CAD build for the part. Positions are in the model's coordinates, mm. A direction names the side the tool comes from. Give positions to 0.01 mm unless a question says otherwise; leave off trailing zeros. Write each loop counter-clockwise with the first axis right and the second up, starting at its lowest first coordinate (ties: lowest second). Pieces come first, ordered by that corner, then holes. Notation, with made-up numbers: (46, 19.25) - (54, 19.25) arc R20 ccw to (54, 48.25) - close; hole circle Ø8 at (-4, -35). An arc over 180 degrees is marked (long way). Write item = value, one per line. Start each with the question number.
```python
from build123d import *

# Parameters (mm, degrees)
SKETCH_1_W             = 55.4
SKETCH_1_H             = 37.5
SKETCH_1_W_2           = 30
SKETCH_1_H_2           = 4
EXTRUDE_1_DEPTH        = 3
SKETCH_2_R             = 1.25
CUT_EXTRUDE_1_DEPTH    = 67.965737508
SKETCH_3_W             = 10
SKETCH_3_H             = 10.5
CUT_EXTRUDE_2_DEPTH    = 67.965737508
FILLET_2_R             = 1
FILLET_3_R             = 2
SKETCH_6_R             = 1.5
CUT_EXTRUDE_4_DEPTH    = 67.965737508
SKETCH_7_R             = 3
CUT_EXTRUDE_5_DEPTH    = 1.8
FILLET_4_R             = 8
SKETCH_10_W            = 31.4
SKETCH_10_H            = 23
CUT_EXTRUDE_6_DEPTH    = 10
FILLET_5_R             = 8
FILLET_6_R             = 2
HOLE_WIZARD_M3_1_D     = 2.5
HOLE_WIZARD_M3_1_DEPTH = 3
HOLE_WIZARD_M3_1_TIP   = 0.751075774


with BuildPart() as part:
    # 草图1 → 凸台-拉伸1 (new body)
    with BuildSketch(Plane(origin=(0, 0, 0), x_dir=(0, 0, -1), z_dir=(1, 0, 0))):
        with Locations((27.7, 18.75)):
            Rectangle(SKETCH_1_W, SKETCH_1_H)
        with Locations((27.7, 34)):
            Rectangle(SKETCH_1_W_2, SKETCH_1_H_2, mode=Mode.SUBTRACT)
    extrude(amount=EXTRUDE_1_DEPTH)

    # 草图2 → 切除-拉伸1 (cut, through all)
    with BuildSketch(Plane(origin=(3, 0, 0), x_dir=(0, 0, -1), z_dir=(1, 0, 0))):
        with Locations((5.2, 21)):
            Circle(SKETCH_2_R)
        with Locations((5.2, 2.5)):
            Circle(SKETCH_2_R)
        with Locations((50.2, 21)):
            Circle(SKETCH_2_R)
        with Locations((50.2, 2.5)):
            Circle(SKETCH_2_R)
    extrude(amount=-CUT_EXTRUDE_1_DEPTH, mode=Mode.SUBTRACT)

    # 草图3 → 切除-拉伸2 (cut, through all)
    with BuildSketch(Plane(origin=(3, 0, 0), x_dir=(0, 0, -1), z_dir=(1, 0, 0))):
        with Locations((5, 32.25)):
            Rectangle(SKETCH_3_W, SKETCH_3_H)
        with Locations((50.4, 32.25)):
            Rectangle(SKETCH_3_W, SKETCH_3_H)
    extrude(amount=-CUT_EXTRUDE_2_DEPTH, mode=Mode.SUBTRACT)

    # 圆角2
    fillet_2_edges = [part.edges().sort_by_distance(p)[0] for p in [
        (1.5, 36, -12.7),
        (1.5, 32, -12.7),
        (1.5, 32, -42.7),
        (1.5, 36, -42.7),
    ]]
    fillet(fillet_2_edges, radius=FILLET_2_R)

    # 圆角3
    fillet_3_edges = [part.edges().sort_by_distance(p)[0] for p in [
        (1.5, 37.5, -10),
        (1.5, 37.5, -45.4),
    ]]
    fillet(fillet_3_edges, radius=FILLET_3_R)

    # 草图6 → 切除-拉伸4 (cut, through all)
    with BuildSketch(Plane.ZY):
        with Locations((-47.4, 13.5)):
            Circle(SKETCH_6_R)
        with Locations((-8, 13.5)):
            Circle(SKETCH_6_R)
    extrude(amount=-CUT_EXTRUDE_4_DEPTH, mode=Mode.SUBTRACT)

    # 草图7 → 切除-拉伸5 (cut)
    with BuildSketch(Plane.ZY):
        with Locations((-47.4, 13.5)):
            Circle(SKETCH_7_R)
        with Locations((-8, 13.5)):
            Circle(SKETCH_7_R)
    extrude(amount=-CUT_EXTRUDE_5_DEPTH, mode=Mode.SUBTRACT)

    # 圆角4
    fillet_4_edges = [part.edges().sort_by_distance(p)[0] for p in [
        (1.5, 27, -10),
        (1.5, 27, -45.4),
    ]]
    fillet(fillet_4_edges, radius=FILLET_4_R)

    # 草图10 → 切除-拉伸6 (cut)
    with BuildSketch(Plane.ZY):
        with Locations((-27.7, 13.5)):
            Rectangle(SKETCH_10_W, SKETCH_10_H)
    extrude(amount=-CUT_EXTRUDE_6_DEPTH, mode=Mode.SUBTRACT)

    # 圆角5
    fillet_5_edges = [part.edges().sort_by_distance(p)[0] for p in [
        (1.5, 25, -12),
        (1.5, 2, -12),
        (1.5, 2, -43.4),
        (1.5, 25, -43.4),
    ]]
    fillet(fillet_5_edges, radius=FILLET_5_R)

    # 圆角6
    fillet_6_edges = [part.edges().sort_by_distance(p)[0] for p in [
        (1.5, 27, -55.4),
        (1.5, 0, -55.4),
        (1.5, 0, 0),
        (1.5, 27, 0),
    ]]
    fillet(fillet_6_edges, radius=FILLET_6_R - 0.0001)  # a hair under: the kernel refuses the full size

    # M3 螺纹孔1
    with Locations(Plane(origin=(0, 21, -50.2), x_dir=(0, 0, -1), z_dir=(-1, 0, 0))):
        with Locations((0, 0), (0, 18.5), (-45, 18.5), (-45, 0)):
            Hole(HOLE_WIZARD_M3_1_D / 2, depth=HOLE_WIZARD_M3_1_DEPTH)
            with Locations((0, 0, -(HOLE_WIZARD_M3_1_DEPTH + HOLE_WIZARD_M3_1_TIP / 2))):  # 118° drill point
                Cone(0, HOLE_WIZARD_M3_1_D / 2, HOLE_WIZARD_M3_1_TIP, mode=Mode.SUBTRACT)


solid = part.part
```
1. Wall check: line 1 along Y through (x, z) = (2.3, -29); line 2 along Y through (x, z) = (2.4, -5.2); line 3 along Z through (x, y) = (1.55, 22) (3 decimals). Give the ranges that are in metal, low to high.
2. Pin check, flat tips, straight feed: pin 1 Ø1.8 at (y, z) = (14.5, -9) entering from -X; pin 2 Ø1.6 at (x, y) = (1, 34) entering from -Z; pin 3 Ø1 at (x, y) = (1, 34) entering from +Z; pin 4 Ø2.5 at (y, z) = (13.5, -8) entering from -X. Stop position of each tip, or through.
3. Cut at C-C (y = 18). Give the cut face in (x, z).
4. Mould opens along Z. For faces 4 (the cylindrical face through (1.48, 26.4, -54.83)), 5 (the cylindrical face through (1.521, 22.719, -14.406)), 6 (the cylindrical face through (1.48, 36.9, -10.57)) say: +Z half, -Z half, draft (parallel to the pull), parting line (faces both ways), or undercut.
5. Cut at A-A (y = 13.5). Give the cut face in (x, z).
6. Cut at D-D (x = 2.5). Count the separate pieces of the cut face and the enclosed holes in it, then the cut area to 3 significant figures.
7. Tool access for faces 1 (the flat face through (0, 27, -27)), 2 (the cylindrical face through (0.89, 10.57, -48.05)), 3 (the cylindrical face through (1.521, 4.406, -14.281)): list every direction of +Z, -Z, +X, -X, +Y, -Y with a clear straight run to the whole face (end or side of a thin tool).
8. Cut at B-B (z = -47.4). Give the cut face in (x, y), then the cut area to 3 significant figures.
Output:
q1.line_1 = 0 to 2, 25 to 32, 36 to 37.5
q1.line_2 = 0 to 1.25, 3.75 to 19.75, 22.25 to 27.67
q1.line_3 = -55.4 to -50.95, -49.45 to -41.645, -13.755 to -5.95, -4.45 to 0
q2.pin_1 = 1.8
q2.pin_2 = -45.61
q2.pin_3 = -9.86
q2.pin_4 = through
q3.outline = (0, -55.4) - (3, -55.4) - (3, -43.34) - (0, -43.34) - close; (0, -12.06) - (3, -12.06) - (3, 0) - (0, 0) - close
q4.face_4 = -Z half
q4.face_5 = undercut
q4.face_6 = +Z half
q5.outline = (0, -55.4) - (3, -55.4) - (3, -48.9) - (1.8, -48.9) - (1.8, -50.4) - (0, -50.4) - close; (0, -44.4) - (1.8, -44.4) - (1.8, -45.9) - (3, -45.9) - (3, -43.4) - (0, -43.4) - close; (0, -12) - (3, -12) - (3, -9.5) - (1.8, -9.5) - (1.8, -11) - (0, -11) - close; (0, -5) - (1.8, -5) - (1.8, -6.5) - (3, -6.5) - (3, 0) - (0, 0) - close
q6.separate_pieces = 1
q6.enclosed_holes = 8
q6.area = 1,070 mm2
q7.face_1 = +Z, -Z, -X, +Y, -Y
q7.face_2 = -X
q7.face_3 = +X, -X
q8.outline = (0, 0) - (3, 0) - (3, 12) - (1.8, 12) - (1.8, 10.5) - (0, 10.5) - close; (0, 16.5) - (1.8, 16.5) - (1.8, 15) - (3, 15) - (3, 29.71) - (0, 29.71) - close
q8.area = 74.7 mm2
